Work out the finished part from the listing and answer in its coordinate system (mm). A direction names the side the tool comes from. Coordinates: 2 decimals unless noted, no trailing zeros. Order: outer loops, then holes, each group sorted by start corner. A loop starts at its lowest first (then second) coordinate and runs counter-clockwise, first axis right, second up. Notation, with made-up numbers: M 15,37 L 55,37 A26 ccw 55,72 Z; hole C -34,58 d10. An arc over 180 degrees is marked long. Write item = value, one per line. Start each with the question number.
Q1. Find section B-B on y = 10.5. Give the vertices of the cut face in (x, z).
Q2. Find section D-D on x = 11. Give the vertices of the cut face in (y, z).
Q3. A tool of negligible diameter and unlimited length cuts with its end or side. For faces 4 (the flat face through (13, 10.8, 1)), 5 (the flat face through (8, 13, 1)), 6 (the flat face through (4.2, 12, 1)), from which of +Z, -Z, +X, -X, +Y, -Y can it reach the whole face along a straight path? Write none if from no direction.
Q4. This flat-tipped pin is pushed along its axis until it touches: P1, Ø0.6, axis at y = 12.5, z = 1, coming from the -X side. Where does it stop, or does it pass through?
Q5. Find section C-C on z = 1.3. Give the vertices of the cut face in (x, y), and give its area (3 significant figures).
Q6. Straight lines are drawn through the part: line 1 along Y through (x, z) = (7.5, 1.15); line 2 along Y through (x, z) = (2, 0.75); line 3 along X through (y, z) = (10, 0.95). For each, find the intervals that lie inside material, in ascending order.
Q7. Determine the mould class of faces 1 (the cylindrical face through (7.15, 12.06, 0.99)), 2 (the flat face through (15, 5, 1)), 3 (the flat face through (7, 0, 1)) for opening direction X: released by +X, released by -X, zero draft, split by the parting line, or undercut.
Q8. Find section A-A on x = 7.5. Give the vertices of the cut face in (y, z), and give its area (3 significant figures).
Autodesk Fusion 360 part; units mm, degrees
sketch "Esquisse1" plane through (0, 0, 0) normal (0, 0, 1) x (1, 0, 0)
  line L0 (0, 0) -> (15, 0)
  line L1 (15, 0) -> (15, 13)
  line L2 (15, 13) -> (0, 13)
  line L3 (0, 13) -> (0, 0)
  line L4 (0, 13) -> (4.2, 13)
  line L5 (4.2, 13) -> (4.2, 10.8)
  line L6 (4.2, 10.8) -> (0, 10.8)
  line L7 (0, 10.8) -> (0, 13)
  line L8 (15, 13) -> (10.8, 13)
  line L9 (10.8, 13) -> (10.8, 10.8)
  line L10 (10.8, 10.8) -> (15, 10.8)
  line L11 (15, 10.8) -> (15, 13)
  line L12 (0, 8) -> (15, 8) construction
  line L13 (7.5, 8) -> (7.5, 13) construction
  circle A0 centre (7.5, 10.5) radius 1.6
  dimension "d1" = 15
  dimension "d2" = 13
  dimension "d3" = 4.2
  dimension "d4" = 2.2
  dimension "d5" = 4.2
  dimension "d6" = 2.2
  dimension "d9" = 5
  dimension "d10" = 3.2
extrude "Extrusion1" add sketch "Esquisse1" along normal blind 2 contours L0 L1 L2 L3 L5 L6 L9 L10
Findings below:
q1.outline = M 0,0 L 5.9,0 L 5.9,2 L 0,2 Z; M 9.1,0 L 15,0 L 15,2 L 9.1,2 Z
q2.outline = M 0,0 L 10.8,0 L 10.8,2 L 0,2 Z
q3.face_4 = +Z, -Z, +X, +Y
q3.face_5 = +Z, -Z, +X, -X, +Y
q3.face_6 = +Z, -Z, -X, +Y
q4.P1 = 4.2
q5.outline = M 0,0 L 15,0 L 15,10.8 L 10.8,10.8 L 10.8,13 L 4.2,13 L 4.2,10.8 L 0,10.8 Z; hole C 7.5,10.5 d3.2
q5.area = 168 mm^2
q6.line_1 = 0 to 8.9, 12.1 to 13
q6.line_2 = 0 to 10.8
q6.line_3 = 0 to 5.98, 9.02 to 15
q7.face_1 = undercut
q7.face_2 = released by +X
q7.face_3 = zero draft
q8.outline = M 0,0 L 8.9,0 L 8.9,2 L 0,2 Z; M 12.1,0 L 13,0 L 13,2 L 12.1,2 Z
q8.area = 19.6 mm^2
